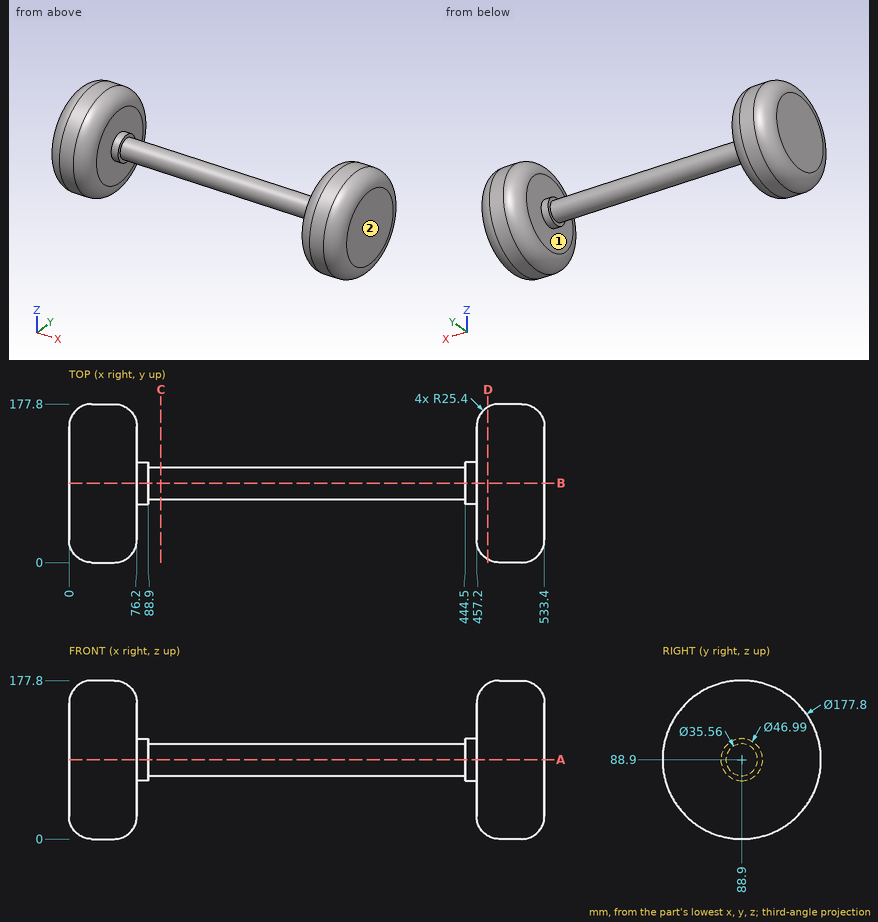
Design review of the part shown in the three views and the two pictorial views. Dimensions are in mm from the part's minimum x, y and z. A direction names the side the tool comes from. Coordinates: 2 decimals unless noted, no trailing zeros. Write each loop counter-clockwise with the first axis right and the second up, starting at its lowest first coordinate (ties: lowest second). Pieces come first, ordered by that corner, then holes.
1) We need section A-A on z = 88.9. State the section outline as (x, y) points (3 decimals), then the cut area to 3 significant figures.
2) We need section D-D on x = 470. State the section outline as (y, z) points.
3) Machinability: for the marked faces 1 and 2, which of the approach directions +Z, -Z, +X, -X, +Y, -Y give a long, thin tool a straight path to every point of the face, cutting with its end or side? Answer none if there is none.
4) We need section C-C on x = 103. State the section outline as (y, z) points, then the cut area to 3 significant figures.
5) To check wall thickness, follow probe 1 along X at (y, z) = (80, 133); probe 2 along Z at (x, y) = (275, 87); probe 3 along X at (y, z) = (19.5, 72). State the ranges of each line that lie inside material, in increasing order.
6) Clearance check with a flat-ended pin moving along its axis: pin 1 Ø3 at (x, y) = (335, 101) entering from +Z. State where the tip first meets the part, or that it passes through.
Answer list:
1. outline: (0, 25.4) arc R25.4 ccw to (25.4, 0) - (50.8, 0) arc R25.4 ccw to (76.2, 25.4) - (76.2, 65.405) - (88.9, 65.405) - (88.9, 71.12) - (444.5, 71.12) - (444.5, 65.405) - (457.2, 65.405) - (457.2, 25.4) arc R25.4 ccw to (482.6, 0) - (508, 0) arc R25.4 ccw to (533.4, 25.4) - (533.4, 152.4) arc R25.4 ccw to (508, 177.8) - (482.6, 177.8) arc R25.4 ccw to (457.2, 152.4) - (457.2, 112.395) - (444.5, 112.395) - (444.5, 106.68) - (88.9, 106.68) - (88.9, 112.395) - (76.2, 112.395) - (76.2, 152.4) arc R25.4 ccw to (50.8, 177.8) - (25.4, 177.8) arc R25.4 ccw to (0, 152.4) - close
1. area: 39,800 mm2
2. outline: circle Ø171.11 at (88.9, 88.9)
3. face 1: none
3. face 2: +Z, -Z, +X, +Y, -Y
4. outline: circle Ø35.56 at (88.9, 88.9)
4. area: 993 mm2
5. probe 1: x = 0 to 76.2, 457.2 to 533.4
5. probe 2: z = 71.22 to 106.58
5. probe 3: x = 1.27 to 74.93, 458.47 to 532.13
6. pin 1: stops at z = 103.17
